```python
from build123d import *

# Parameters (mm, degrees)
SKETCH3_W           = 8.1
SKETCH3_H           = 2.8
SKETCH3_R           = 0.45
BOSS_EXTRUDE1_DEPTH = 5
SKETCH4_R           = 0.45
BOSS_EXTRUDE4_DEPTH = 9
SKETCH7_W           = 1
SKETCH7_H           = 4
CUT_EXTRUDE2_DEPTH  = 0.5


with BuildPart() as part:
    # Sketch3 → Boss-Extrude1 (new body)
    with BuildSketch(Plane(origin=(0, 0, 0), x_dir=(1, 0, 0), z_dir=(0, 1, 0))):
        Rectangle(SKETCH3_W, SKETCH3_H)
        with Locations((2.5, 0)):
            Circle(SKETCH3_R, mode=Mode.SUBTRACT)
        with Locations((-2.5, 0)):
            Circle(SKETCH3_R, mode=Mode.SUBTRACT)
        Circle(SKETCH3_R, mode=Mode.SUBTRACT)
    extrude(amount=-BOSS_EXTRUDE1_DEPTH)

    # Sketch4 → Boss-Extrude4 (add)
    with BuildSketch(Plane.XZ.offset(5)):
        Polygon((4.05, -0.65), (3.3, -1.4), (-3.3, -1.4), (-4.05, -0.65), (-4.05, 1.4), (4.05, 1.4), align=None)
        with Locations((2.5, 0)):
            Circle(SKETCH4_R, mode=Mode.SUBTRACT)
        Circle(SKETCH4_R, mode=Mode.SUBTRACT)
        with Locations((-2.5, 0)):
            Circle(SKETCH4_R, mode=Mode.SUBTRACT)
    extrude(amount=BOSS_EXTRUDE4_DEPTH)

    # Sketch7 → Cut-Extrude2 (cut)
    with BuildSketch(Plane.XY.offset(1.4)):
        with Locations((-3.75, -7)):
            Rectangle(SKETCH7_W, SKETCH7_H)
        with Locations((3.75, -7)):
            Rectangle(SKETCH7_W, SKETCH7_H)
        with Locations((-1.25, -7)):
            Rectangle(SKETCH7_W, SKETCH7_H)
        with Locations((1.25, -7)):
            Rectangle(SKETCH7_W, SKETCH7_H)
    extrude(amount=-CUT_EXTRUDE2_DEPTH, mode=Mode.SUBTRACT)


solid = part.part
```
The model under review builds one solid part; all positions refer to its coordinate system, in mm. A direction names the side the tool comes from. Give positions to 0.01 mm unless a question says otherwise; leave off trailing zeros. Write each loop counter-clockwise with the first axis right and the second up, starting at its lowest first coordinate (ties: lowest second). Pieces come first, ordered by that corner, then holes. Notation, with made-up numbers: (68, 13.25) -> (94, 13.25) arc R21 ccw to (94, 32.25) -> close; hole circle Ø11 at (74.5, 50). An arc over 180 degrees is marked (long way). Answer in a Markdown table with one row per item.
1) For L1, parallel to X at y = -1.05, z = 0; L2, parallel to X at y = -10.25, z = 0.35; L3, parallel to Z at x = -2.5, y = -8.5, list the stretches that pass through material, from the lowest coordinate up. Write a range as [from, to].
Worked answers:
| item | result |
|---|---|
| L1 | [-4.05, -2.95], [-2.05, -0.45], [0.45, 2.05], [2.95, 4.05] |
| L2 | [-4.05, -2.78], [-2.22, -0.28], [0.28, 2.22], [2.78, 4.05] |
| L3 | [-1.4, -0.45], [0.45, 1.4] |
2) Add section A-A on x = 0. State the section outline as (y, z) points, plus the area to 3 significant figures.
Worked answers:
| item | result |
|---|---|
| outline | (-14, -1.4) -> (0, -1.4) -> (0, -0.45) -> (-14, -0.45) -> close; (-14, 0.45) -> (0, 0.45) -> (0, 1.4) -> (-14, 1.4) -> close |
| area | 26.6 mm² |
3) Add section D-D on z = -1.05. State the section outline as (x, y) points, plus the area to 3 significant figures.
Worked answers:
| item | result |
|---|---|
| outline | (-4.05, -5) -> (-3.65, -5) -> (-3.65, -14) -> (3.65, -14) -> (3.65, -5) -> (4.05, -5) -> (4.05, 0) -> (-4.05, 0) -> close |
| area | 106 mm² |
4) Mouldability with a two-part tool opening along X and no side actions: class faces 3 (the flat face through (0, -7, 1.4)), 4 (the flat face through (1, -7, 0.9)), 5 (the flat face through (-4.05, -7, 0)) as +X half, -X half, draft (parallel to the pull), parting line (faces both ways), or undercut.
Worked answers:
| item | result |
|---|---|
| face 3 | draft |
| face 4 | undercut |
| face 5 | -X half |
5) Add section C-C on y = -6.25. State the section outline as (x, z) points, plus the area to 3 significant figures.
Worked answers:
| item | result |
|---|---|
| outline | (-4.05, -0.65) -> (-3.3, -1.4) -> (3.3, -1.4) -> (4.05, -0.65) -> (4.05, 0.9) -> (3.25, 0.9) -> (3.25, 1.4) -> (1.75, 1.4) -> (1.75, 0.9) -> (0.75, 0.9) -> (0.75, 1.4) -> (-0.75, 1.4) -> (-0.75, 0.9) -> (-1.75, 0.9) -> (-1.75, 1.4) -> (-3.25, 1.4) -> (-3.25, 0.9) -> (-4.05, 0.9) -> close; hole circle Ø0.9 at (-2.5, 0); hole circle Ø0.9 at (0, 0); hole circle Ø0.9 at (2.5, 0) |
| area | 18.4 mm² |
6) Clearance check with flat-ended pins moving along their axes: P1, Ø0.6, axis at x = 4, y = -7, coming from the +Z side; P2, Ø0.6, axis at y = -7, z = 1.5, coming from the -X side. State where each tip first meets the part, or that it passes through.
Worked answers:
| item | result |
|---|---|
| P1 | z = 0.9 |
| P2 | x = -3.25 |
7) Tool access review of faces 1 (the flat face through (-1, -7, 0.9)), 2 (the flat face through (0, -7, -1.4)): name each direction out of +Z, -Z, +X, -X, +Y, -Y from which nothing blocks a thin tool from reaching the whole face with its end or side.
Worked answers:
| item | result |
|---|---|
| face 1 | +Z |
| face 2 | -Z, +X, -X, +Y, -Y |
8) Add section B-B on z = 0. State the section outline as (x, y) points.
Worked answers:
| item | result |
|---|---|
| outline | (-4.05, -14) -> (-2.95, -14) -> (-2.95, 0) -> (-4.05, 0) -> close; (-2.05, -14) -> (-0.45, -14) -> (-0.45, 0) -> (-2.05, 0) -> close; (0.45, -14) -> (2.05, -14) -> (2.05, 0) -> (0.45, 0) -> close; (2.95, -14) -> (4.05, -14) -> (4.05, 0) -> (2.95, 0) -> close |
